Read the model definition and answer for the solid it produces. Units are mm, in the model's axes. Face numbers are marked on the shaded views. A direction names the side the tool comes from. Coordinates: 2 decimals unless noted, no trailing zeros. Loops run counter-clockwise (first coordinate to the right, second up) from the corner with the lowest first, then second, coordinate; pieces in that order, holes last.
Q1. The mould has two halves that part along Y. Classify the marked faces 5, 6 and 7: pulls with the +Y half, pulls with the -Y half, needs draft (parallel to the pull), parting line crosses it, or undercut.
Q2. Flat-ended cylindrical pins translate along their axes: P1, Ø2, axis at x = 1, y = 8, coming from the -Z side; P2, Ø0.7, axis at x = 4, z = 0, coming from the -Y side; P3, Ø1.5, axis at x = 7.5, y = 8.5, coming from the +Z side. Find the tip coordinate at first contact, or state that the pin passes through.
Q3. Section A-A (x = 0) is taken. Give the vertices of the cut face in (y, z), then the cut area to 3 significant figures.
Q4. Straight lines are drawn through the part: line 1 (Y direction, x = -14, z = 4.5); line 2 (Z direction, x = 0, y = 9.25). For each, find the intervals that lie inside material, in ascending order.
Q5. Section B-B (z = 0) is taken. Give the vertices of the cut face in (x, y).
Q6. Which of the six approach directions +Z, -Z, +X, -X, +Y, -Y give full straight-line access (tool end or side, diameter ignored) to the marked faces 1, 2, 3 and 4?
from build123d import *

# Parameters (mm, degrees)
EXTRUDE_1_DEPTH     = 10.2
SKETCH_3_R          = 17.5
EXTRUDE_2_DEPTH     = 2
EXTRUDE_START       = 2
SKETCH_4_R          = 17.5
EXTRUDE_3_DEPTH     = 2
CUT_EXTRUDE_4_DEPTH = 10
CUT_EXTRUDE_START   = -4.2
SKETCH_6_R          = 4.05
CUT_EXTRUDE_5_DEPTH = 4.2
CHAMFER_1_SIZE      = 0.5
CHAMFER_2_SIZE      = 0.5


with BuildPart() as part:
    # Эскиз2 → Вытянуть1 (new body)
    with BuildSketch(Plane(origin=(0, 0, 0), x_dir=(1, 0, 0), z_dir=(0, 1, 0))):
        with BuildLine():
            Line((-0.9, 14.171450173), (-1.326328648, 15.342778507))
            ThreePointArc((-1.326328648, 15.342778507), (-2.409090762, 15.210400445), (-3.479765796, 15.00170757))
            Line((-3.479765796, 15.00170757), (-3.523268074, 13.755965327))
            ThreePointArc((-3.523268074, 13.755965327), (-4.38804132, 13.505002531), (-5.235169803, 13.199734737))
            Line((-5.235169803, 13.199734737), (-6.002592803, 14.181991385))
            ThreePointArc((-6.002592803, 14.181991385), (-6.991453696, 13.721500473), (-7.945236519, 13.192164972))
            Line((-7.945236519, 13.192164972), (-7.60165412, 11.993950752))
            ThreePointArc((-7.60165412, 11.993950752), (-8.346550583, 11.48804132), (-9.05788471, 10.935937298))
            Line((-9.05788471, 10.935937298), (-10.091281352, 11.632972134))
            ThreePointArc((-10.091281352, 11.632972134), (-10.88944443, 10.88944443), (-11.632972134, 10.091281352))
            Line((-11.632972134, 10.091281352), (-10.935937298, 9.05788471))
            ThreePointArc((-10.935937298, 9.05788471), (-11.48804132, 8.346550583), (-11.993950752, 7.60165412))
            Line((-11.993950752, 7.60165412), (-13.192164972, 7.945236519))
            ThreePointArc((-13.192164972, 7.945236519), (-13.721500473, 6.991453696), (-14.181991385, 6.002592803))
            Line((-14.181991385, 6.002592803), (-13.199734737, 5.235169803))
            ThreePointArc((-13.199734737, 5.235169803), (-13.505002531, 4.38804132), (-13.755965327, 3.523268074))
            Line((-13.755965327, 3.523268074), (-15.00170757, 3.479765796))
            ThreePointArc((-15.00170757, 3.479765796), (-15.210400445, 2.409090762), (-15.342778507, 1.326328648))
            Line((-15.342778507, 1.326328648), (-14.171450173, 0.9))
            ThreePointArc((-14.171450173, 0.9), (-14.2, 0), (-14.171450173, -0.9))
            Line((-14.171450173, -0.9), (-15.342778507, -1.326328648))
            ThreePointArc((-15.342778507, -1.326328648), (-15.210400445, -2.409090762), (-15.00170757, -3.479765796))
            Line((-15.00170757, -3.479765796), (-13.755965327, -3.523268074))
            ThreePointArc((-13.755965327, -3.523268074), (-13.505002531, -4.38804132), (-13.199734737, -5.235169803))
            Line((-13.199734737, -5.235169803), (-14.181991385, -6.002592803))
            ThreePointArc((-14.181991385, -6.002592803), (-13.721500473, -6.991453696), (-13.192164972, -7.945236519))
            Line((-13.192164972, -7.945236519), (-11.993950752, -7.60165412))
            ThreePointArc((-11.993950752, -7.60165412), (-11.48804132, -8.346550583), (-10.935937298, -9.05788471))
            Line((-10.935937298, -9.05788471), (-11.632972134, -10.091281352))
            ThreePointArc((-11.632972134, -10.091281352), (-10.88944443, -10.88944443), (-10.091281352, -11.632972134))
            Line((-10.091281352, -11.632972134), (-9.05788471, -10.935937298))
            ThreePointArc((-9.05788471, -10.935937298), (-8.346550583, -11.48804132), (-7.60165412, -11.993950752))
            Line((-7.60165412, -11.993950752), (-7.945236519, -13.192164972))
            ThreePointArc((-7.945236519, -13.192164972), (-6.991453696, -13.721500473), (-6.002592803, -14.181991385))
            Line((-6.002592803, -14.181991385), (-5.235169803, -13.199734737))
            ThreePointArc((-5.235169803, -13.199734737), (-4.38804132, -13.505002531), (-3.523268074, -13.755965327))
            Line((-3.523268074, -13.755965327), (-3.479765796, -15.00170757))
            ThreePointArc((-3.479765796, -15.00170757), (-2.409090762, -15.210400445), (-1.326328648, -15.342778507))
            Line((-1.326328648, -15.342778507), (-0.9, -14.171450173))
            ThreePointArc((-0.9, -14.171450173), (0, -14.2), (0.9, -14.171450173))
            Line((0.9, -14.171450173), (1.326328648, -15.342778507))
            ThreePointArc((1.326328648, -15.342778507), (2.409090762, -15.210400445), (3.479765796, -15.00170757))
            Line((3.479765796, -15.00170757), (3.523268074, -13.755965327))
            ThreePointArc((3.523268074, -13.755965327), (4.38804132, -13.505002531), (5.235169803, -13.199734737))
            Line((5.235169803, -13.199734737), (6.002592803, -14.181991385))
            ThreePointArc((6.002592803, -14.181991385), (6.991453696, -13.721500473), (7.945236519, -13.192164972))
            Line((7.945236519, -13.192164972), (7.60165412, -11.993950752))
            ThreePointArc((7.60165412, -11.993950752), (8.346550583, -11.48804132), (9.05788471, -10.935937298))
            Line((9.05788471, -10.935937298), (10.091281352, -11.632972134))
            ThreePointArc((10.091281352, -11.632972134), (10.88944443, -10.88944443), (11.632972134, -10.091281352))
            Line((11.632972134, -10.091281352), (10.935937298, -9.05788471))
            ThreePointArc((10.935937298, -9.05788471), (11.48804132, -8.346550583), (11.993950752, -7.60165412))
            Line((11.993950752, -7.60165412), (13.192164972, -7.945236519))
            ThreePointArc((13.192164972, -7.945236519), (13.721500473, -6.991453696), (14.181991385, -6.002592803))
            Line((14.181991385, -6.002592803), (13.199734737, -5.235169803))
            ThreePointArc((13.199734737, -5.235169803), (13.505002531, -4.38804132), (13.755965327, -3.523268074))
            Line((13.755965327, -3.523268074), (15.00170757, -3.479765796))
            ThreePointArc((15.00170757, -3.479765796), (15.210400445, -2.409090762), (15.342778507, -1.326328648))
            Line((15.342778507, -1.326328648), (14.171450173, -0.9))
            ThreePointArc((14.171450173, -0.9), (14.2, 0), (14.171450173, 0.9))
            Line((14.171450173, 0.9), (15.342778507, 1.326328648))
            ThreePointArc((15.342778507, 1.326328648), (15.210400445, 2.409090762), (15.00170757, 3.479765796))
            Line((15.00170757, 3.479765796), (13.755965327, 3.523268074))
            ThreePointArc((13.755965327, 3.523268074), (13.505002531, 4.38804132), (13.199734737, 5.235169803))
            Line((13.199734737, 5.235169803), (14.181991385, 6.002592803))
            ThreePointArc((14.181991385, 6.002592803), (13.721500473, 6.991453696), (13.192164972, 7.945236519))
            Line((13.192164972, 7.945236519), (11.993950752, 7.60165412))
            ThreePointArc((11.993950752, 7.60165412), (11.48804132, 8.346550583), (10.935937298, 9.05788471))
            Line((10.935937298, 9.05788471), (11.632972134, 10.091281352))
            ThreePointArc((11.632972134, 10.091281352), (10.88944443, 10.88944443), (10.091281352, 11.632972134))
            Line((10.091281352, 11.632972134), (9.05788471, 10.935937298))
            ThreePointArc((9.05788471, 10.935937298), (8.346550583, 11.48804132), (7.60165412, 11.993950752))
            Line((7.60165412, 11.993950752), (7.945236519, 13.192164972))
            ThreePointArc((7.945236519, 13.192164972), (6.991453696, 13.721500473), (6.002592803, 14.181991385))
            Line((6.002592803, 14.181991385), (5.235169803, 13.199734737))
            ThreePointArc((5.235169803, 13.199734737), (4.38804132, 13.505002531), (3.523268074, 13.755965327))
            Line((3.523268074, 13.755965327), (3.479765796, 15.00170757))
            ThreePointArc((3.479765796, 15.00170757), (2.409090762, 15.210400445), (1.326328648, 15.342778507))
            Line((1.326328648, 15.342778507), (0.9, 14.171450173))
            ThreePointArc((0.9, 14.171450173), (0, 14.2), (-0.9, 14.171450173))
        make_face()
    extrude(amount=EXTRUDE_1_DEPTH)

    # Эскиз3 → Вытянуть2 (add)
    with BuildSketch(Plane(origin=(0, 10.2, 0), x_dir=(1, 0, 0), z_dir=(0, 1, 0))):
        with Locations(Location((0, 0, 0), (0, 0, 270))):
            Circle(SKETCH_3_R)
    extrude(amount=EXTRUDE_2_DEPTH)

    # Эскиз4 → Вытянуть3 (add)
    with BuildSketch(Plane.XZ.offset(EXTRUDE_START)):
        with Locations(Location((0, 0, 0), (0, 0, 90))):
            Circle(SKETCH_4_R)
    extrude(amount=-EXTRUDE_3_DEPTH)

    # Эскиз5 → Вытянуть4 (cut)
    with BuildSketch(Plane(origin=(0, 12.2, 0), x_dir=(1, 0, 0), z_dir=(0, 1, 0))):
        with BuildLine():
            Line((3.45, -2.121320344), (3.45, 2.121320344))
            ThreePointArc((3.45, 2.121320344), (-2.863782464, 2.863782464), (-2.121320344, -3.45))
            Line((-2.121320344, -3.45), (2.121320344, -3.45))
            ThreePointArc((2.121320344, -3.45), (2.863782464, -2.863782464), (3.45, -2.121320344))
        make_face()
    extrude(amount=-CUT_EXTRUDE_4_DEPTH, mode=Mode.SUBTRACT)

    # Эскиз6 → Вытянуть5 (cut)
    with BuildSketch(Plane.XZ.offset(2).offset(CUT_EXTRUDE_START)):
        with Locations(Location((0, 0, 0), (0, 0, 58.413661903))):
            Circle(SKETCH_6_R)
    extrude(amount=CUT_EXTRUDE_5_DEPTH, mode=Mode.SUBTRACT)

    # Фаска1
    chamfer_1_edges = [part.edges().sort_by_distance(p)[0] for p in [
        (-2.863782464, 12.2, -2.863782464),
        (0, 12.2, 3.45),
        (2.863782464, 12.2, 2.863782464),
        (3.45, 12.2, 0),
    ]]
    chamfer(chamfer_1_edges, length=CHAMFER_1_SIZE)

    # Фаска2
    chamfer_2_edges = [part.edges().sort_by_distance(p)[0] for p in [
        (-2.121320344, -2, -3.45),
    ]]
    chamfer(chamfer_2_edges, length=CHAMFER_2_SIZE)


solid = part.part
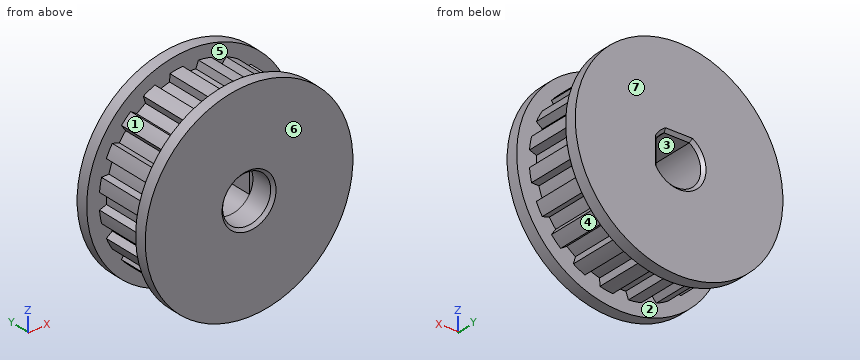
Numbers:
1. face 5: undercut
1. face 6: pulls with the -Y half
1. face 7: pulls with the +Y half
2. P1: stops at z = -15.34
2. P2: stops at y = -1.8
2. P3: stops at z = 13.84
3. outline: (-2, -17.5) - (0, -17.5) - (0, -14.2) - (10.2, -14.2) - (10.2, -17.5) - (12.2, -17.5) - (12.2, -4.55) - (11.7, -4.05) - (-1.5, -4.05) - (-2, -4.55) - close; (-2, 4.55) - (-1.5, 4.05) - (2.2, 4.05) - (2.2, 3.45) - (11.7, 3.45) - (12.2, 3.95) - (12.2, 17.5) - (10.2, 17.5) - (10.2, 14.2) - (0, 14.2) - (0, 17.5) - (-2, 17.5) - close
3. area: 320 mm2
4. line 1: y = -2 to 0, 10.2 to 12.2
4. line 2: z = -14.2 to -4.05, 3.45 to 14.2
5. outline: (-17.5, -2) - (-4.55, -2) - (-4.05, -1.5) - (-4.05, 11.7) - (-4.55, 12.2) - (-17.5, 12.2) - (-17.5, 10.2) - (-14.2, 10.2) - (-14.2, 0) - (-17.5, 0) - close; (3.45, 2.2) - (4.05, 2.2) - (4.05, -1.5) - (4.55, -2) - (17.5, -2) - (17.5, 0) - (14.2, 0) - (14.2, 10.2) - (17.5, 10.2) - (17.5, 12.2) - (3.95, 12.2) - (3.45, 11.7) - close
6. face 1: +Z, -X
6. face 2: none
6. face 3: +Y, -Y
6. face 4: -Z, +X
